from build123d import *

# Parameters (mm, degrees)
SKETCH1_R           = 7.672873739
BOSS_EXTRUDE1_DEPTH = 25.4
SKETCH2_W           = 15.345747478
SKETCH2_H           = 12.7
BOSS_EXTRUDE2_DEPTH = 1.820422808
BOSS_EXTRUDE3_DEPTH = 25.4
SKETCH5_W           = 0.549916313
SKETCH5_H           = 38.1
BOSS_EXTRUDE4_DEPTH = 25.4
SKETCH6_W           = 25.4
SKETCH6_H           = 6.473300788
BOSS_EXTRUDE5_DEPTH = 25.4


with BuildPart() as part:
    # Sketch1 → Boss-Extrude1 (new body)
    with BuildSketch(Plane.XY):
        Circle(SKETCH1_R)
    extrude(amount=BOSS_EXTRUDE1_DEPTH)

    # Sketch2 → Boss-Extrude2 (add)
    with BuildSketch(Plane(origin=(0, 0, 0), x_dir=(-1, 0, 0), z_dir=(0, 0, -1))):
        with Locations((0, 6.35)):
            Rectangle(SKETCH2_W, SKETCH2_H)
    extrude(amount=-BOSS_EXTRUDE2_DEPTH)

    # Sketch4 → Boss-Extrude3 (add)
    with BuildSketch(Plane(origin=(0, 0, 0), x_dir=(-1, 0, 0), z_dir=(0, 0, -1))):
        Polygon((-31.75, 12.7), (-31.75, 22.935187234), (31.75, 22.935187234), (31.75, 12.7), (7.672873739, 12.7), (-7.672873739, 12.7), align=None)
    extrude(amount=-BOSS_EXTRUDE3_DEPTH)

    # Sketch5 → Boss-Extrude4 (add)
    with BuildSketch(Plane(origin=(0, 0, 0), x_dir=(-1, 0, 0), z_dir=(0, 0, -1))):
        with Locations((31.475041844, 41.985187234)):
            Rectangle(SKETCH5_W, SKETCH5_H)
        with Locations((-31.475041844, 41.985187234)):
            Rectangle(SKETCH5_W, SKETCH5_H)
    extrude(amount=-BOSS_EXTRUDE4_DEPTH)

    # Sketch6 → Boss-Extrude5 (add)
    with BuildSketch(Plane(origin=(0, 0, 0), x_dir=(-1, 0, 0), z_dir=(0, 0, -1))):
        with Locations((19.05, 64.271837628)):
            Rectangle(SKETCH6_W, SKETCH6_H)
        with Locations((-19.05, 64.271837628)):
            Rectangle(SKETCH6_W, SKETCH6_H)
    extrude(amount=-BOSS_EXTRUDE5_DEPTH)


solid = part.part
The model under review builds one solid part; all positions refer to its coordinate system, in mm. A direction names the side the tool comes from. Give positions to 0.01 mm unless a question says otherwise; leave off trailing zeros. Order: outer loops, then holes, each group sorted by start corner. A loop starts at its lowest first (then second) coordinate and runs counter-clockwise, first axis right, second up. Notation, with made-up numbers: M 60.5,2.25 L 96.5,2.25 A11 ccw 96.5,23.25 Z; hole C 13,-40 d7. An arc over 180 degrees is marked long. One line per question, with ' | ' between items. Start each with the question number.
1) Wall thickness on L1, parallel to Y at x = 24.5, z = 19.25; L2, parallel to X at y = 30, z = 11.25; L3, parallel to X at y = 0.5, z = 14: over which ranges is each line inside the solid? List them lowest first. Write a range as from..to.
2) Clearance check with flat-ended pins moving along their axes: P1, Ø7.5, axis at x = 24, z = 12, coming from the -Y side; P2, Ø6, axis at x = -24.5, y = 27.5, coming from the -Z side; P3, Ø4, axis at x = -4, y = 7.5, coming from the +Z side; P4, Ø7.5, axis at x = 8, z = 7.5, coming from the -Y side. State where each tip first meets the part, or that it passes through.
3) For faces 1 (the face through (31.2, 42, 13)), 2 (the face through (-6.35, 64, 13)), 3 (the face through (7.673, 6, 1)), list the 3-axis set-ups (+Z, -Z, +X, -X, +Y, -Y) from which the entire face can be reached by the end or side of a thin tool; tool diameter is ignored.
4) Consider section A-A, the plane z = 9.25. Give the boundary of the cut face in (x, y).
5) Mouldability with a two-part tool opening along Y and no side actions: class faces 4 (the face through (-19, 61.035, 13)), 5 (the face through (6.35, 64, 13)), 6 (the face through (19, 67.508, 13)) as pulls with the +Y half, pulls with the -Y half, needs draft (parallel to the pull), parting line crosses it, or undercut.
6) Consider section C-C, the plane x = 20. Give the boundary of the cut face in (y, z).
7) Consider section D-D, the plane x = 0.5. Give the boundary of the cut face in (y, z), then the cut area to 3 significant figures.
8) Consider section B-B, the plane y = 42.5. Give the boundary of the cut face in (x, z).
Found:
1) L1: y = 12.7..22.94, 61.04..67.51 | L2: x = -31.75..-31.2, 31.2..31.75 | L3: x = -7.66..7.66
2) P1: stops at y = 12.7 | P2: passes through | P3: stops at z = 25.4 | P4: stops at y = -6.39
3) face 1: +Z, -Z | face 2: +Z, -Z, +Y | face 3: +Z, -Z, +X, -Y
4) outline: M -31.75,12.7 L 31.75,12.7 L 31.75,67.51 L 6.35,67.51 L 6.35,61.04 L 31.2,61.04 L 31.2,22.94 L -31.2,22.94 L -31.2,61.04 L -6.35,61.04 L -6.35,67.51 L -31.75,67.51 Z; C 0,0 d15.35
5) face 4: undercut | face 5: needs draft | face 6: pulls with the +Y half
6) outline: M 12.7,0 L 22.94,0 L 22.94,25.4 L 12.7,25.4 Z; M 61.04,0 L 67.51,0 L 67.51,25.4 L 61.04,25.4 Z
7) outline: M -7.66,0 L 22.94,0 L 22.94,25.4 L 12.7,25.4 L 12.7,1.82 L 7.66,1.82 L 7.66,25.4 L -7.66,25.4 Z | area: 658 mm²
8) outline: M -31.75,0 L -31.2,0 L -31.2,25.4 L -31.75,25.4 Z; M 31.2,0 L 31.75,0 L 31.75,25.4 L 31.2,25.4 Z
